The model under review builds one solid part; all positions refer to its coordinate system, in mm. Face numbers are marked on the shaded views. A direction names the side the tool comes from. Round coordinates to 2 decimals unless told otherwise and drop trailing zeros. Order: outer loops, then holes, each group sorted by start corner. A loop starts at its lowest first (then second) coordinate and runs counter-clockwise, first axis right, second up. Notation, with made-up numbers: M 77.5,2 L 135.5,2 A7 ccw 135.5,7 Z; hole C 17,22 d8. An arc over 180 degrees is marked long. Use a Markdown table: item, result. Add a question column.
1. Consider section A-A on x = 0. State the section outline as (y, z) points, then the cut area to 3 significant figures.
2. The part is to be moulded in two halves that separate along X. For the marked faces 1, 2, 3 and 4, say which applies: +X half, -X half, draft (parallel to the pull), parting line (faces both ways), or undercut.
3. Insertion check: P1, Ø3.5, axis at x = -1.5, z = 4, coming from the +Y side; P2, Ø1, axis at y = -5, z = 1.5, coming from the +X side; P3, Ø5.5, axis at x = -0.5, z = 4.5, coming from the -Y side. Each pin has a flat end and moves straight along its axis. Give the tip position at first contact, or say it passes through.
4. For the marked faces 5, 6 and 7, list the 3-axis set-ups (+Z, -Z, +X, -X, +Y, -Y) from which the entire face can be reached by the end or side of a thin tool; tool diameter is ignored.
5. To check wall thickness, follow probe 1 along Y at (x, z) = (0, 3.5); probe 2 along Z at (x, y) = (-10.5, 7.5); probe 3 along X at (y, z) = (-3.25, 8.25). State the ranges of each line that lie inside material, in increasing order.
6. Consider section B-B on z = 2.75. State the section outline as (x, y) points.
Autodesk Inventor part; units mm, degrees
ref_plane "YZ Plane" through (0, 0, 0) normal (1, 0, 0) x (0, 1, 0)
ref_plane "XZ Plane" through (0, 0, 0) normal (0, 1, 0) x (-1, 0, 0)
ref_plane "XY Plane" through (0, 0, 0) normal (0, 0, 1) x (1, 0, 0)
sketch "草图1" plane through (0, 0, 0) normal (0, 0, 1) x (1, 0, 0)
  circle A0 centre (0, 0) radius 15
  dimension "d0" = 30
extrude "拉伸1" add sketch "草图1" along normal blind 2
sketch "草图2" plane through (0, 0, 2) normal (0, 0, 1) x (1, 0, 0)
  line L0 (5.7735, -10) -> (-5.7735, -10)
  line L1 (-5.7735, -10) -> (-11.547, 0)
  line L2 (-11.547, 0) -> (-5.7735, 10)
  line L3 (-5.7735, 10) -> (5.7735, 10)
  line L4 (5.7735, 10) -> (11.547, 0)
  line L5 (11.547, 0) -> (5.7735, -10)
  line L6 (0, 0) -> (0, 1.986)
  point P0 (0, 10)
  dimension "d3" = 1.986
  dimension "d4" = 20
extrude "拉伸2" add sketch "草图2" along normal blind 8
sketch "草图3" plane through (0, 0, 10) normal (0, 0, 1) x (1, 0, 0)
  circle A0 centre (0, 0) radius 5
  dimension "d7" = 10
extrude "拉伸3" cut sketch "草图3" against normal through all
thread "螺纹1"
fillet "圆角1" radius 1 13 edges at (-15, 0, 2) (-5.7735, 10, 6) (-11.547, 0, 6) (-5.7735, -10, 6) (11.547, 0, 6) (5.7735, 10, 6) (5.7735, -10, 6) (8.6603, -5, 10) (8.6603, 5, 10) (0, 10, 10) (-8.6603, 5, 10) (-8.6603, -5, 10) (0, -10, 10)
chamfer "倒角1" distance 0.25 angle 45 1 edges at (-5, 0, 10)
chamfer "倒角2" distance 0.25 angle 45 1 edges at (-5, 0, 0)
properties part number "主动轮固定螺帽"
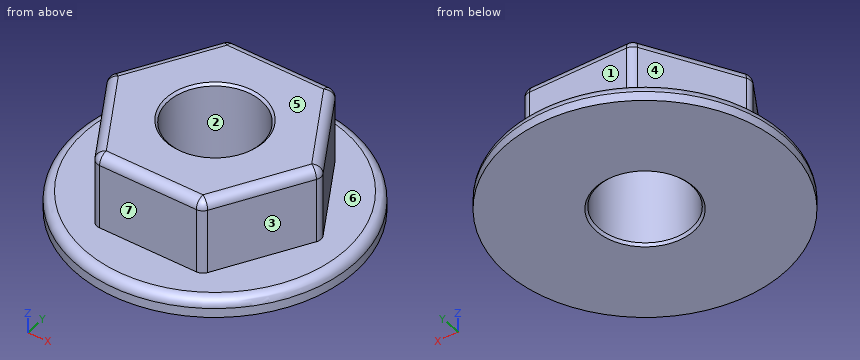
Answer block:
| question | item | result |
|---|---|---|
| 1 | outline | M -15,0 L -5.25,0 L -5,0.25 L -5,9.75 L -5.25,10 L -9,10 A1 ccw -10,9 L -10,2 L -14,2 A1 ccw -15,1 Z; M 5,0.25 L 5.25,0 L 15,0 L 15,1 A1 ccw 14,2 L 10,2 L 10,9 A1 ccw 9,10 L 5.25,10 L 5,9.75 Z |
| 1 | area | 119 mm^2 |
| 2 | face 1 | draft |
| 2 | face 2 | undercut |
| 2 | face 3 | +X half |
| 2 | face 4 | -X half |
| 3 | P1 | y = 10 |
| 3 | P2 | x = 14.26 |
| 3 | P3 | y = -14.65 |
| 4 | face 5 | +Z, +X, -X, +Y, -Y |
| 4 | face 6 | +Z |
| 4 | face 7 | +Z, +X, -X, -Y |
| 5 | probe 1 | -10 to -5, 5 to 10 |
| 5 | probe 2 | 0 to 2 |
| 5 | probe 3 | -9.67 to -3.8, 3.8 to 9.67 |
| 6 | outline | M -11.26,-0.5 L -6.06,-9.5 A1 ccw -5.2,-10 L 5.2,-10 A1 ccw 6.06,-9.5 L 11.26,-0.5 A1 ccw 11.26,0.5 L 6.06,9.5 A1 ccw 5.2,10 L -5.2,10 A1 ccw -6.06,9.5 L -11.26,0.5 A1 ccw Z; hole C 0,0 d10 |
